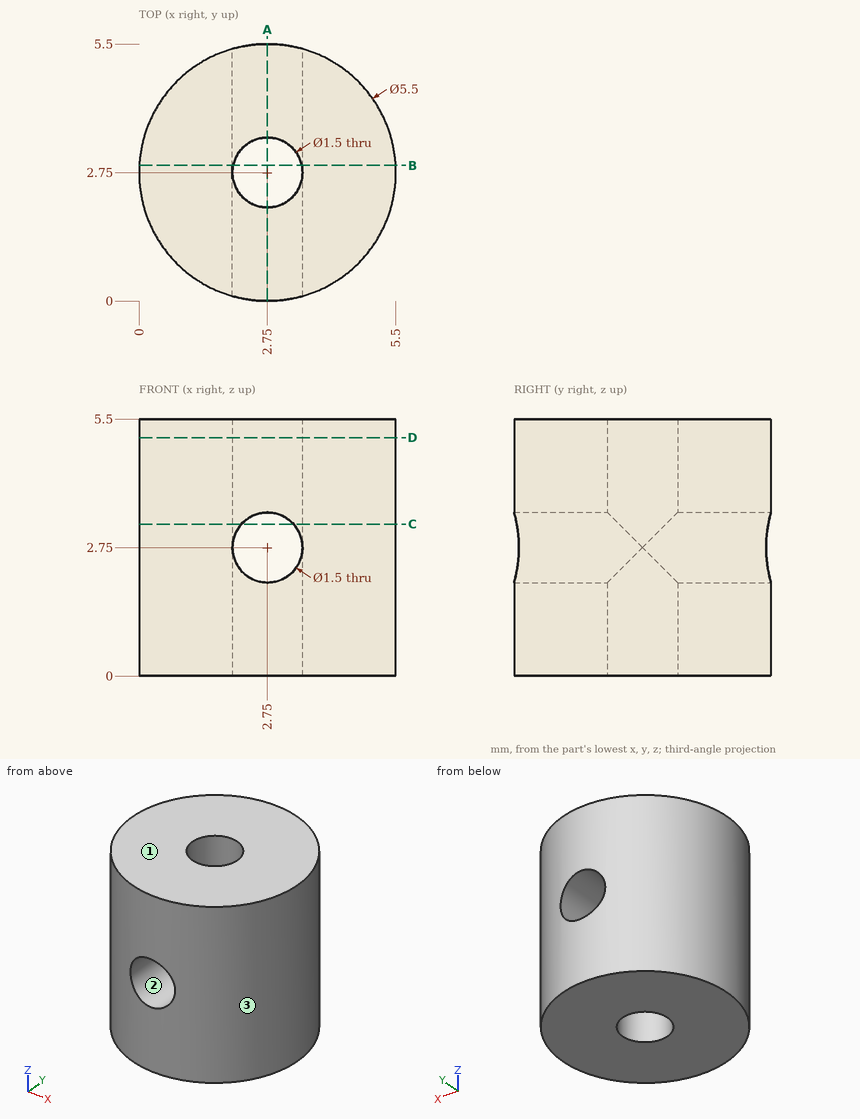
Here's the drawing with two shaded views (mm, measured from the low corner). I have some questions. Coordinates: 2 decimals unless noted, no trailing zeros. Write each loop counter-clockwise with the first axis right and the second up, starting at its lowest first coordinate (ties: lowest second). Pieces come first, ordered by that corner, then holes.
Item 1: If I drill on line 1 (Y direction, x = 2.75, z = 1); line 2 (Z direction, x = 3, y = 5.3), over which ranges is the centre line in solid material (lowest first)?
Item 2: I want a section at C-C on z = 3.25. Write out the boundary of the cut face in (x, y), and give its area (3 significant figures).
Item 3: Will these pins go through, and if not, where does the flat tip stop? pin 1 (0.9 mm diameter, centred on x = 2.75, y = 2.75, fed in from -Z); pin 2 (3 mm diameter, centred on y = 4.5, z = 1.5, fed in from +X).
Item 4: If we mould it in two halves opening along X, with no side actions, what happens to the marked faces 1, 2 and 3? For each: +X half, -X half, draft (parallel to the pull), parting line (faces both ways), or undercut.
Item 5: I want a section at A-A on x = 2.75. Write out the boundary of the cut face in (y, z).
Item 6: I want a section at B-B on y = 2.9. Write out the boundary of the cut face in (x, z), and give its area (3 significant figures).
Item 7: I want a section at D-D on z = 5.1. Write out the boundary of the cut face in (x, y), and give its area (3 significant figures).
Findings below:
1. line 1: y = 0 to 2, 3.5 to 5.5
1. line 2: z = 0 to 2.04, 3.46 to 5.5
2. outline: (2.19, 0.06) - (2.19, 2.25) arc R0.75 cw to (2.19, 3.25) - (2.19, 5.44) arc R2.75 ccw to start; (3.31, 0.06) arc R2.75 ccw to (3.31, 5.44) - (3.31, 3.25) arc R0.75 cw to (3.31, 2.25) - close
2. area: 17.4 mm2
3. pin 1: passes through
3. pin 2: stops at x = 5.49
4. face 1: draft
4. face 2: undercut
4. face 3: parting line
5. outline: (0, 0) - (2, 0) - (2, 2) - (0, 2) - close; (0, 3.5) - (2, 3.5) - (2, 5.5) - (0, 5.5) - close; (3.5, 0) - (5.5, 0) - (5.5, 2) - (3.5, 2) - close; (3.5, 3.5) - (5.5, 3.5) - (5.5, 5.5) - (3.5, 5.5) - close
6. outline: (0, 0) - (2.02, 0) - (2.02, 2.6) arc R0.75 cw to (2.02, 2.9) - (2.02, 5.5) - (0, 5.5) - close; (3.48, 0) - (5.5, 0) - (5.5, 5.5) - (3.48, 5.5) - (3.48, 2.9) arc R0.75 cw to (3.48, 2.6) - close
6. area: 22.1 mm2
7. outline: circle Ø5.5 at (2.75, 2.75); hole circle Ø1.5 at (2.75, 2.75)
7. area: 22.0 mm2
